The model under review builds one solid part; all positions refer to its coordinate system, in mm. A direction names the side the tool comes from. Coordinates: 2 decimals unless noted, no trailing zeros. Order: outer loops, then holes, each group sorted by start corner. A loop starts at its lowest first (then second) coordinate and runs counter-clockwise, first axis right, second up. Notation, with made-up numbers: (-32.5, 26.25) -> (-20.5, 26.25) arc R13 cw to (-20.5, 31.25) -> close; hole circle Ø11 at (51.25, -14). An arc over 180 degrees is marked (long way). Use one line per item in the form item = value.
Autodesk Inventor part; units mm, degrees
ref_plane "YZ Plane" through (0, 0, 0) normal (1, 0, 0) x (0, 1, 0)
ref_plane "XZ Plane" through (0, 0, 0) normal (0, 1, 0) x (-1, 0, 0)
ref_plane "XY Plane" through (0, 0, 0) normal (0, 0, 1) x (1, 0, 0)
sketch "BackwithHoles" plane through (0, 0, 0) normal (0, 1, 0) x (-1, 0, 0)
  line L0 (0, 0) -> (25, 0)
  line L1 (25, 0) -> (25, 60)
  line L2 (25, 60) -> (0, 60)
  line L3 (0, 60) -> (0, 0)
  circle A0 centre (12.5, 47.5) radius 3
  circle A1 centre (12.5, 17.5) radius 3
  dimension "d8" = 25
  dimension "d9" = 60
  dimension "d10" = 6
  dimension "d11" = 6
  dimension "d12" = 12.5
  dimension "d13" = 12.5
  dimension "d14" = 12.5
  dimension "d15" = 17.5
extrude "Extrusion1" add sketch "BackwithHoles" along normal blind 4
sketch "Bottom" plane through (0, 4, 0) normal (0, 1, 0) x (1, 0, 0)
  line L0 (0, -60) -> (0, 0)
  line L1 (0, 0) -> (-25, 0)
  line L2 (0, -5) -> (-25, -5)
  line L3 (-25, -5) -> (-25, 0)
  line L4 (-25, 0) -> (0, 0)
  line L5 (0, 0) -> (0, -5)
  dimension "d18" = 5
extrude "Extrusion2" add sketch "Bottom" along normal blind 15
sketch "HolesonBottom" plane through (-25, 4, 5) normal (0, 0, 1) x (1, 0, 0)
  circle A0 centre (17.5, 7.5) radius 2.5
  circle A1 centre (5, 7.5) radius 2.5
  line L0 (25, 0) -> (25, 15)
  line L1 (0, 0) -> (0, 15)
  line L2 (0, 0) -> (25, 0)
  point P0 (25, -4)
  dimension "d21" = 5
  dimension "d22" = 5
  dimension "d23" = 7.5
  dimension "d24" = 5
  dimension "d25" = 7.5
  dimension "d26" = 7.5
  dimension "d27" = 12.5
hole "Hole1" at (-7.5, 11.5, 5) at (-20, 11.5, 5) direction (0, 0, -1) diameter 5.86 end through all
sketch "TopSquare" plane through (0, 4, 0) normal (0, 1, 0) x (1, 0, 0)
  line L0 (-20, -55) -> (-5, -55)
  line L1 (-5, -55) -> (-5, -40)
  line L2 (-5, -40) -> (-20, -40)
  line L3 (-20, -40) -> (-20, -55)
  line L4 (-25, -60) -> (0, -60)
  line L5 (0, -60) -> (0, -5)
  point P0 (0, 0)
  dimension "d35" = 5
  dimension "d36" = 15
  dimension "d37" = 15
  dimension "d38" = 5
extrude "Extrusion3" cut sketch "TopSquare" against normal blind 3
sketch "BottomSquare" plane through (0, 4, 0) normal (0, 1, 0) x (1, 0, 0)
  line L0 (-20, -25) -> (-5, -25)
  line L1 (-5, -25) -> (-5, -10)
  line L2 (-5, -10) -> (-20, -10)
  line L3 (-20, -10) -> (-20, -25)
  line L4 (0, -60) -> (0, -5)
  line L5 (-20, -40) -> (-5, -40)
  point P0 (0, 0)
  point P1 (-20, -40)
  dimension "d41" = 15
  dimension "d42" = 15
  dimension "d43" = 5
  dimension "d44" = 30
extrude "Extrusion4" cut sketch "BottomSquare" against normal blind 3
sketch "BottomExtrusion" plane through (0, 19, 0) normal (0, 1, 0) x (1, 0, 0)
  line L0 (0, 0) -> (-25, 0)
  line L1 (-25, 0) -> (-25, -5)
  line L2 (0, 0) -> (-25, 0)
  line L3 (-25, 0) -> (-25, -5)
  line L4 (-25, -5) -> (0, -5)
  line L5 (0, -5) -> (0, 0)
extrude "Extrusion7" add sketch "BottomExtrusion" along normal blind 23
sketch "BottomExteriorExtrusion" plane through (0, 0, 60) normal (1, 0, 0) x (0, 0, -1)
  line L0 (55, 42) -> (60, 42)
  line L1 (60, 0) -> (55, 0)
  line L2 (55, 0) -> (55, 42)
  line L3 (55, 42) -> (60, 42)
  line L4 (60, 42) -> (60, 0)
extrude "Extrusion8" add sketch "BottomExteriorExtrusion" along normal blind 12
sketch "ContainingWall" plane through (-25, 4, 5) normal (0, 0, 1) x (1, 0, 0)
  line L0 (37, -4) -> (37, 38)
  line L1 (0, 38) -> (37, 38)
  line L2 (37, 15) -> (32, 15)
  line L3 (32, 15) -> (32, 38)
  line L4 (32, 38) -> (37, 38)
  line L5 (37, 38) -> (37, 15)
  point P0 (25, -4)
  dimension "d56" = 5
  dimension "d57" = 23
extrude "Extrusion9" add sketch "ContainingWall" along normal blind 45
sketch "ContainingWallExtension" plane through (0, 42, 0) normal (0, 1, 0) x (1, 0, 0)
  line L0 (12, 0) -> (12, -50)
  line L1 (7, -50) -> (12, -50)
  line L2 (12, -50) -> (7, -50)
  line L3 (-25, -5) -> (7, -5)
  line L4 (7, -50) -> (7, -5)
  line L5 (7, -5) -> (-25, -5)
  line L6 (-25, 0) -> (12, 0)
  line L7 (-25, -5) -> (-25, 0)
  line L8 (-25, 0) -> (12, 0)
  line L9 (12, 0) -> (12, -50)
  point P0 (0, 0)
extrude "Extrusion10" add sketch "ContainingWallExtension" along normal blind 12
sketch "AnteriorBottomExtension" plane through (-25, 0, 0) normal (-1, 0, 0) x (0, 0, 1)
  line L0 (5, 0) -> (0, 0)
  line L1 (0, 0) -> (0, 54)
  line L2 (0, 0) -> (0, 54)
  line L3 (5, 19) -> (5, 54)
  line L4 (0, 54) -> (5, 54)
  line L5 (5, 19) -> (5, 0)
  line L6 (5, 54) -> (5, 0)
  line L7 (5, 0) -> (0, 0)
extrude "Extrusion11" add sketch "AnteriorBottomExtension" along normal blind 5
properties part number "Slider" material "Wood (Maple)"
Item 1: We need section C-C (x = -21.5). Write out the cut boundary in (y, z).
Results found:
outline = (0, 0) -> (8.98, 0) -> (8.98, 5) -> (4, 5) -> (4, 60) -> (0, 60) -> close; (14.02, 0) -> (54, 0) -> (54, 5) -> (14.02, 5) -> close
Item 2: We need section A-A (z = 32.5). Write out the cut boundary in (x, y).
Results found:
outline = (-25, 0) -> (0, 0) -> (0, 4) -> (-25, 4) -> close; (7, 19) -> (12, 19) -> (12, 54) -> (7, 54) -> close
Item 3: We need section B-B (y = 11.5). Write out the cut boundary in (x, z), plus the area to 3 significant figures.
Results found:
outline = (-30, 0) -> (-22.93, 0) -> (-22.93, 5) -> (-30, 5) -> close; (-17.07, 0) -> (-10.43, 0) -> (-10.43, 5) -> (-17.07, 5) -> close; (-4.57, 0) -> (12, 0) -> (12, 5) -> (-4.57, 5) -> close
area = 151 mm²
Item 4: Draft analysis for pull direction X (two halves, no side actions). For faces 1 (the face through (-13, 0, 30)), 2 (the face through (-25, 2, 33)), 3 (the face through (-5, 3, 48)), 4 (the face through (-10.1, 0.5, 19.3)), state which applies: released by +X, released by -X, zero draft, split by the parting line, or undercut.
Results found:
face_1 = zero draft
face_2 = released by -X
face_3 = undercut
face_4 = undercut
Item 5: We need section D-D (z = 47.5). Write out the cut boundary in (x, y), plus the area to 3 significant figures.
Results found:
outline = (-25, 0) -> (-15.5, 0) -> (-15.5, 1) -> (-20, 1) -> (-20, 4) -> (-25, 4) -> close; (-9.5, 0) -> (0, 0) -> (0, 4) -> (-5, 4) -> (-5, 1) -> (-9.5, 1) -> close; (7, 19) -> (12, 19) -> (12, 54) -> (7, 54) -> close
area = 224 mm²
Item 6: To check wall thickness, follow L1, parallel to X at y = 11.5, z = 2; L2, parallel to Y at x = -7.5, z = 1.4; L3, parallel to X at y = 0.5, z = 17.5. State the ranges of each line that lie inside material, in increasing order. Write a range as from..to.
Results found:
L1 = -30..-22.93, -17.07..-10.43, -4.57..12
L2 = 0..8.57, 14.43..54
L3 = -25..-15.5, -9.5..0
Item 7: Clearance check with flat-ended pins moving along their axes: pin 1 (4 mm diameter, centred on y = 21, z = 10.5, fed in from -X); pin 2 (2.5 mm diameter, centred on y = 2, z = 14.5, fed in from -X); pin 3 (4 mm diameter, centred on x = 9, y = 28, fed in from +Z). State where each tip first meets the part, or that it passes through.
Results found:
pin_1 = 7
pin_2 = -25
pin_3 = 50
Item 8: Tool access review of faces 5 (the face through (7, 36, 28)), 6 (the face through (-13, 1, 14)), 7 (the face through (0, 2, 33)): name each direction out of +Z, -Z, +X, -X, +Y, -Y from which nothing blocks a thin tool from reaching the whole face with its end or side.
Results found:
face_5 = +Z, -X, +Y, -Y
face_6 = +Y
face_7 = +Z, +X, +Y, -Y
